Can you work these out from the model? Positions are in its coordinate system, mm. Face numbers are marked on the shaded views. A direction names the side the tool comes from. Give positions to 0.01 mm unless a question says otherwise; leave off trailing zeros. Order: outer loops, then holes, each group sorted by start corner. A loop starts at its lowest first (then second) coordinate and runs counter-clockwise, first axis right, second up. Notation, with made-up numbers: (15, 86.25) - (23, 86.25) arc R27 ccw to (23, 115.25) - close; hole circle Ø4 at (50.5, -24). An arc over 180 degrees is marked (long way). Answer as CSV lines item,"result".
Autodesk Inventor part; units mm, degrees
ref_plane "Work Plane2" through (0, 200, 0) normal (0, -1, 0) x (1, 0, 0)
ref_plane "YZ Plane" through (0, 0, 0) normal (1, 0, 0) x (0, 1, 0)
ref_plane "XZ Plane" through (0, 0, 0) normal (0, 1, 0) x (-1, 0, 0)
sketch "Sketch1" plane through (0, 0, 0) normal (0, 0, 1) x (1, 0, 0)
  line L0 (0, 0) -> (0, 15)
  line L1 (0, 850) -> (-280, 850)
  line L2 (-280, 850) -> (-280, 595)
  line L3 (-280, 0) -> (0, 0)
  arc A0 (-280, 324) -> (-280, 284) centre (-274.1667, 304) ccw
  line L4 (-280, 0) -> (-278, 0)
  line L5 (-278, 0) -> (-278, 15)
  line L6 (-278, 15) -> (0, 15)
  arc A1 (-280, 595) -> (-280, 555) centre (-274.1667, 575) ccw
  line L7 (-278, 15) -> (-280, 15)
  line L8 (-280, 15) -> (-280, 0)
  line L9 (0, 15) -> (0, 850)
  line L10 (-279, 15) -> (-279, 284.96)
  line L11 (-279, 849) -> (-1, 849)
  line L12 (-1, 849) -> (-1, 15)
  line L13 (-279, 849) -> (-279, 850)
  line L14 (-279, 16) -> (-1, 16)
  line L15 (-1, 16) -> (0, 16)
  arc A2 (-279.72, 594.04) -> (-279.72, 555.96) centre (-274.1667, 575) ccw
  line L16 (-279.72, 555.96) -> (-279, 555.96)
  line L17 (-279.72, 594.04) -> (-279, 594.04)
  line L18 (-279, 594.04) -> (-279, 849)
  line L19 (-279, 555.96) -> (-279, 594.04)
  line L20 (-280, 556.0439) -> (-280, 555)
  line L21 (-280, 593.9561) -> (-280, 556.0439)
  line L22 (-280, 595) -> (-280, 593.9561)
  line L23 (-280, 555) -> (-280, 324)
  arc A3 (-279.72, 323.04) -> (-280, 285.0439) centre (-274.1667, 304) ccw
  line L24 (-279.72, 323.04) -> (-279, 323.04)
  line L25 (-279.72, 284.96) -> (-279, 284.96)
  arc A4 (-280, 285.0439) -> (-279.72, 284.96) centre (-274.1667, 304) ccw
  line L26 (-280, 284) -> (-280, 15)
  line L27 (-279, 284.96) -> (-279, 555.96)
  line L28 (-280, 322.9561) -> (-280, 284)
  line L29 (-280, 324) -> (-280, 322.9561)
  point P0 (-295, 304)
  point P1 (-295, 575)
  dimension "d0" = 850
  dimension "d1" = 280
  dimension "d2" = 40
  dimension "d3" = 15
  dimension "d5" = 2
  dimension "d6" = 15
  dimension "d7" = 284
  dimension "d8" = 40
  dimension "d9" = 15
  dimension "d10" = 255
  dimension "d14" = 1
  dimension "d15" = 1
  dimension "d16" = 1
  dimension "d17" = 1
revolve "Revolution1" add sketch "Sketch1" angle 360 about axis through (0, 15, 0) along (0, 1, 0) contours L6 L12 L15 L9 | L3 L8 L7 L5 | L6 L7 L10 L14 L12 | L26 L28 A4 L25 L10 L7 | L13 L18 L17 A2 L22 L2 L1 | A0 L29 A3 L28 | L23 L20 A2 L16 L27 L24 A3 L29 | L22 A2 L20 A1
ref_plane "Work Plane2" through (0, 200, 0) normal (0, -1, 0) x (1, 0, 0)
sketch "Sketch5" plane through (0, 200, 0) normal (0, -1, 0) x (1, 0, 0)
  circle A0 centre (0, 0) radius 280
  circle A1 centre (0, 0) radius 280
  circle A2 centre (0, 0) radius 280
  circle A3 centre (0, 0) radius 280
  circle A4 centre (0, 0) radius 290
  line L0 (0, 0) -> (-276.1822, 39.5525)
  line L1 (0, 0) -> (276.1822, 39.5525)
  line L2 (0, 0) -> (0, 290)
  circle A5 centre (0, 0) radius 279
  line L3 (-276.1822, 39.5525) -> (-287.0711, 41.1119)
  line L4 (276.1822, 39.5525) -> (287.0711, 41.1119)
  circle A6 centre (0, 0) radius 390
  line L5 (-287.0711, 41.1119) -> (-386.0611, 55.2884)
  line L6 (276.1822, 39.5525) -> (386.0611, 55.2884)
  line L7 (0, 279) -> (0, 390)
  dimension "d29" = 10
  dimension "d30" = 81.85
  dimension "d31" = 163.7
  dimension "d32" = 100
extrude "Extrusion2" cut sketch "Sketch5" against normal blind 480 contours L3 A4 L2 A0 | A0 L2 A5 L3 | L5 A6 L7 A4 keep common part
properties part number "Fass"
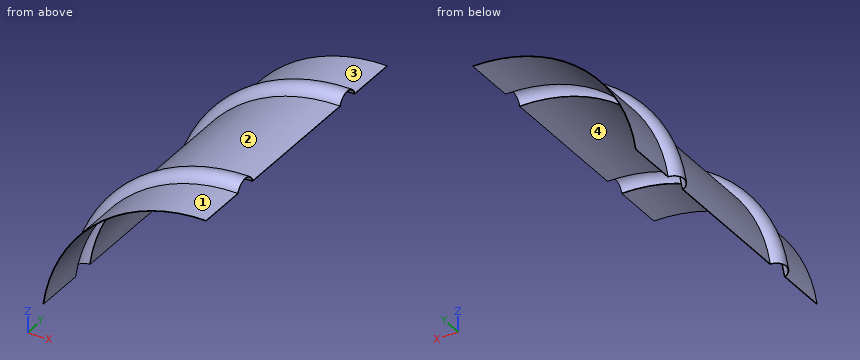
1) I want a section at A-A on y = 416. Write out the boundary of the cut face in (x, z).
Answer block:
outline,"(-277.17, 39.69) - (-276.18, 39.55) arc R279 cw to (0, 279) - (0, 280) arc R280 ccw to start"
2) If we mould it in two halves opening along Y, with no side actions, what happens to the marked faces 1 and 2? For each: +Y half, -Y half, draft (parallel to the pull), parting line (faces both ways), or undercut.
Answer block:
face 1,"draft"
face 2,"undercut"
3) I need wall thicknesses on line 1 along Y through (x, z) = (-217, 195); line 2 along Z through (x, y) = (-166, 541); line 3 along Z through (x, y) = (-151, 401). Which ranges of each line are inside material? Lowest first, please. Write a range as [from, to].
Answer block:
line 1,"[292.82, 294.81], [313.19, 315.18], [563.82, 565.81], [584.19, 586.18]"
line 2,"[224.24, 225.49]"
line 3,"[234.61, 235.79]"
4) I'm going to push flat-ended pins straight in: P1, Ø6, axis at x = -191.5, y = 549.5, coming from the -Z side; P2, Ø2, axis at y = 529.5, z = 137, coming from the +X side; P3, Ø5, axis at y = 420, z = 175.5, coming from the +X side. Where does each tip first touch, or does it pass through?
Answer block:
P1,"z = 200.03"
P2,"x = -242.48"
P3,"x = -214.84"
5) Which directions (+Z, -Z, +X, -X, +Y, -Y) give clear straight access to the entire face, cutting with the end or side of a thin tool? Please do the marked faces 3 and 4.
Answer block:
face 3,"+Z, -X, +Y"
face 4,"-Z, +X, +Y, -Y"
